Autodesk Inventor part; units mm, degrees
ref_plane "YZ Plane" through (0, 0, 0) normal (1, 0, 0) x (0, 1, 0)
ref_plane "XZ Plane" through (0, 0, 0) normal (0, 1, 0) x (-1, 0, 0)
ref_plane "XY Plane" through (0, 0, 0) normal (0, 0, 1) x (1, 0, 0)
sketch "Sketch1" plane through (0, 0, 0) normal (0, 1, 0) x (-1, 0, 0)
  circle A0 centre (0, 0) radius 4
  dimension "d0" = 8
extrude "Extrusion1" add sketch "Sketch1" along normal blind 22.5
sketch "Sketch2" plane through (0, 22.5, 0) normal (0, 1, 0) x (1, 0, 0)
  point P0 (0, 0)
  point P1 (0, 0)
hole "Hole1" at (0, 22.5, 0) direction (0, -1, 0) diameter 3.4 end through all
ref_plane "Work Plane1" through (0, 11.25, 0) normal (0, 1, 0) x (1, 0, 0)
mirror "Mirror1" about plane through (0, 11.25, 0) normal (0, 1, 0) of "Hole1"
ref_plane "Work Plane2" through (0, 5, 0) normal (0, -1, 0) x (1, 0, 0)
sketch "Sketch3" plane through (0, 5, 0) normal (0, -1, 0) x (1, 0, 0)
  circle A0 centre (0, 0) radius 2.75
  line L0 (-2.75, 1.5877) -> (0, 3.1754)
  line L1 (0, 3.1754) -> (2.75, 1.5877)
  line L2 (2.75, 1.5877) -> (2.75, -1.5877)
  line L3 (2.75, -1.5877) -> (0, -3.1754)
  line L4 (0, -3.1754) -> (-2.75, -1.5877)
  line L5 (-2.75, -1.5877) -> (-2.75, 1.5877)
  point P0 (-2.75, 0)
  dimension "d11" = 5.5
extrude "Extrusion2" cut sketch "Sketch3" against normal blind 2.48
mirror "Mirror2" about plane through (0, 11.25, 0) normal (0, 1, 0) of "Extrusion2"
properties part number "rod mount motor  for print"
For this review, take the finished solid that the model builds, in its own axes (mm). A direction names the side the tool comes from. Coordinates: 2 decimals unless noted, no trailing zeros. Loops run counter-clockwise (first coordinate to the right, second up) from the corner with the lowest first, then second, coordinate; pieces in that order, holes last. Notation, with made-up numbers: (-4.5, -11) -> (26.5, -11) arc R37 ccw to (26.5, 28) -> close; hole circle Ø6 at (60.25, -36.5). An arc over 180 degrees is marked (long way). Return JSON: item names as keys, results as strings. Group by question number.
(1) Consider section A-A, the plane z = 0. Give the boundary of the cut face in (x, y), plus the area to 3 significant figures.
(2) Tool access review of faces 1 (the cylindrical face through (1.66, 2.46, -0.37)), 2 (the flat face through (2.75, 6, 0)): name each direction out of +Z, -Z, +X, -X, +Y, -Y from which nothing blocks a thin tool from reaching the whole face with its end or side.
(3) Consider section C-C, the plane z = -2.25. Give the boundary of the cut face in (x, y).
(4) For pin 1 Ø2 at (x, z) = (0, 0) entering from +Y; pin 2 Ø0.7 at (y, z) = (17, 0.5) entering from +X, all flat-tipped, find the tip position at first contact; note any pin that passes through.
(5) Consider section B-B, the plane x = 0.75. Give the boundary of the cut face in (y, z), plus the area to 3 significant figures.
(6) Consider section D-D, the plane x = -2. Give the boundary of the cut face in (y, z).
(7) Mouldability with a two-part tool opening along X and no side actions: class faces 3 (the flat face through (-1.394, 6.223, 2.37)), 4 (the flat face through (-2, 0, 0)) as pulls with the +X half, pulls with the -X half, needs draft (parallel to the pull), parting line crosses it, or undercut.
(8) To check wall thickness, follow L1, parallel to Y at x = 1.5, z = -1; L2, parallel to Z at x = 0, y = 4; L3, parallel to Z at x = -1, y = 2.25. State the ranges of each line that lie inside material, in increasing order.
Results below:
{
 "1": {"outline": "(-4, 0) -> (-1.7, 0) -> (-1.7, 5) -> (-2.75, 5) -> (-2.75, 7.48) -> (-1.7, 7.48) -> (-1.7, 15.02) -> (-2.75, 15.02) -> (-2.75, 17.5) -> (-1.7, 17.5) -> (-1.7, 22.5) -> (-4, 22.5) -> close; (1.7, 0) -> (4, 0) -> (4, 22.5) -> (1.7, 22.5) -> (1.7, 17.5) -> (2.75, 17.5) -> (2.75, 15.02) -> (1.7, 15.02) -> (1.7, 7.48) -> (2.75, 7.48) -> (2.75, 5) -> (1.7, 5) -> close", "area": "93.1 mm2"},
 "2": {"face 1": "+Y, -Y", "face 2": "none"},
 "3": {"outline": "(-3.31, 0) -> (3.31, 0) -> (3.31, 22.5) -> (-3.31, 22.5) -> close; hole (-1.6, 5) -> (1.6, 5) -> (1.6, 7.48) -> (-1.6, 7.48) -> close; hole (-1.6, 15.02) -> (1.6, 15.02) -> (1.6, 17.5) -> (-1.6, 17.5) -> close"},
 "4": {"pin 1": "passes through", "pin 2": "stops at x = 4"},
 "5": {"outline": "(0, -3.93) -> (22.5, -3.93) -> (22.5, -1.53) -> (17.5, -1.53) -> (17.5, -2.74) -> (15.02, -2.74) -> (15.02, -1.53) -> (7.48, -1.53) -> (7.48, -2.74) -> (5, -2.74) -> (5, -1.53) -> (0, -1.53) -> close; (0, 1.53) -> (5, 1.53) -> (5, 2.74) -> (7.48, 2.74) -> (7.48, 1.53) -> (15.02, 1.53) -> (15.02, 2.74) -> (17.5, 2.74) -> (17.5, 1.53) -> (22.5, 1.53) -> (22.5, 3.93) -> (0, 3.93) -> close", "area": "96.1 mm2"},
 "6": {"outline": "(0, -3.46) -> (22.5, -3.46) -> (22.5, 3.46) -> (0, 3.46) -> close; hole (5, -2.02) -> (7.48, -2.02) -> (7.48, 2.02) -> (5, 2.02) -> close; hole (15.02, -2.02) -> (17.5, -2.02) -> (17.5, 2.02) -> (15.02, 2.02) -> close"},
 "7": {"face 3": "undercut", "face 4": "needs draft"},
 "8": {"L1": "y = 0 to 5, 7.48 to 15.02, 17.5 to 22.5", "L2": "z = -4 to -1.7, 1.7 to 4", "L3": "z = -3.87 to -1.37, 1.37 to 3.87"}
}
